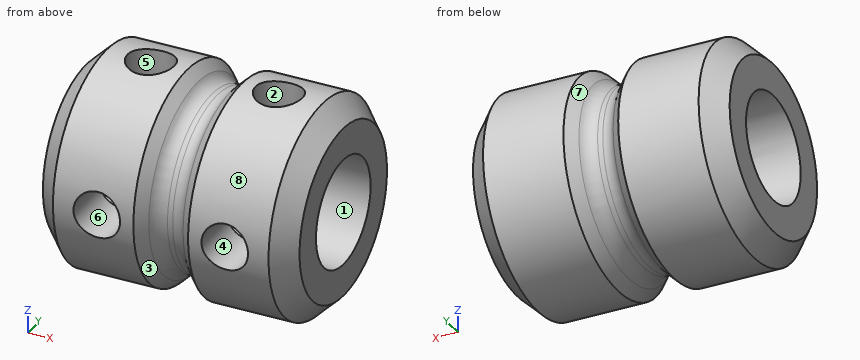
```python
from build123d import *

# Parameters (mm, degrees)
F0_R      = 7.874
F0_R_2    = 3.96875
F1_DEPTH  = 19.05
F2_SIZE2  = 1.524
F2_SIZE   = 1.524
F5_D      = 3.4544
F5_DEPTH  = 9.49325
F5_START  = 0.9537702
F5_TIP    = 1.0378064612
F8_D      = 3.4544
F8_DEPTH  = 9.4996
F8_START  = 0.9537702
F8_TIP    = 1.0378064612
F11_SIZE2 = 0.762
F11_SIZE  = 0.762


# Not quite as in the source:
# - a fillet or chamfer that OpenCascade refuses, or shapes differently, is made with other operations: its cross-section is extruded or revolved along the edge and cut away or added


with BuildPart() as f1:
    # F0 (on Right) → F1 (new body)
    with BuildSketch(Plane.YZ):
        Circle(F0_R)
        Circle(F0_R_2, mode=Mode.SUBTRACT)
    extrude(amount=F1_DEPTH)

    # F2
    f2_edges = [f1.edges().sort_by_distance(p)[0] for p in [
        (19.05, -7.874, 0),
        (0, -7.874, 0),
    ]]
    chamfer(f2_edges, length=F2_SIZE, length2=F2_SIZE2)

    # F5
    # its depths count from where the whole tool has entered the part; down to there all is cleared
    with Locations(Plane.XY.offset(8.636).offset(-F5_START)):
        with Locations((4.7752, 0), (14.2748, 0)):
            Hole(F5_D / 2, depth=F5_DEPTH)
            with Locations((0, 0, -(F5_DEPTH + F5_TIP / 2))):  # 118° drill point
                Cone(0, F5_D / 2, F5_TIP, mode=Mode.SUBTRACT)

    # F8
    # its depths count from where the whole tool has entered the part; down to there all is cleared
    with Locations(Plane.XZ.offset(8.636).offset(-F8_START)):
        with Locations((4.7752, 0), (14.2748, 0)):
            Hole(F8_D / 2, depth=F8_DEPTH)
            with Locations((0, 0, -(F8_DEPTH + F8_TIP / 2))):  # 118° drill point
                Cone(0, F8_D / 2, F8_TIP, mode=Mode.SUBTRACT)

    # F9 (on Front) → F10 (revolve, cut)
    with BuildSketch(Plane.XZ):
        Polygon((10.795, 8.9425863698), (9.525, 8.9425863698), (8.255, 8.9425863698), (8.255, 6.5122395754), (10.795, 6.5122395754), align=None)
    revolve(axis=Axis((-2.5821820018, 0, 0), (-1, 0, 0)), mode=Mode.SUBTRACT)

    # F11
    f11_edges = [f1.edges().sort_by_distance(p)[0] for p in [
        (8.255, -7.874, 0),
        (10.795, -7.874, 0),
    ]]
    chamfer(f11_edges, length=F11_SIZE, length2=F11_SIZE2)

    # F12: fillet of radius 1.27 on 2 edges, made by hand

    # F12_s1 → F12_t2 (revolve)
    with BuildSketch(Plane.XZ):
        with BuildLine():
            ThreePointArc((8.255, 7.112), (8.7166107711, 6.6722611385), (9.3337395013, 6.5122395754))
            Line((9.3337395013, 6.5122395754), (9.3337395013, 6.4868395754))
            Line((9.3337395013, 6.4868395754), (8.255, 6.4868395754))
            Line((8.255, 6.4868395754), (8.2296, 6.5122395754))
            ThreePointArc((8.2296, 6.5122395754), (8.2296, 6.8121197877), (8.23342521, 7.0985952085))
            Line((8.23342521, 7.0985952085), (8.255, 7.112))
        make_face()
    revolve(axis=Axis((8.255, 0, 0), (-1, 0, 0)))

    # F12_s3 → F12_t4 (revolve)
    with BuildSketch(Plane.XZ):
        with BuildLine():
            ThreePointArc((9.7162604987, 6.5122395754), (10.3333892289, 6.6722611385), (10.795, 7.112))
            Line((10.795, 7.112), (10.81657479, 7.0985952085))
            ThreePointArc((10.81657479, 7.0985952085), (10.8204, 6.8121197877), (10.8204, 6.5122395754))
            Line((10.8204, 6.5122395754), (10.795, 6.4868395754))
            Line((10.795, 6.4868395754), (9.7162604987, 6.4868395754))
            Line((9.7162604987, 6.4868395754), (9.7162604987, 6.5122395754))
        make_face()
    revolve(axis=Axis((10.795, 0, 0), (-1, 0, 0)))


solid = f1.part
```
Model file for the job. Use its own axes, mm. Face numbers are marked on the shaded views. A direction names the side the tool comes from. Give positions to 0.01 mm unless a question says otherwise; leave off trailing zeros. Order: outer loops, then holes, each group sorted by start corner. A loop starts at its lowest first (then second) coordinate and runs counter-clockwise, first axis right, second up.
1) 3-axis set-ups, long thin cutter, end or side, ignore diameter. For the marked faces 5, 6, 7 and 8: which of +Z, -Z, +X, -X, +Y, -Y reach the whole face in a straight line?
2) Saw through at A-A, the plane z = 0. Count the separate pieces of the cut face and the enclosed holes in it, then the cut area to 3 significant figures.
3) Mould opens along Z. For the marked faces 1, 2, 3 and 4 say: +Z half, -Z half, draft (parallel to the pull), parting line (faces both ways), or undercut.
4) Saw through at D-D, the plane x = 16.75. Write the cut outline in (y, z).
5) Pin check, flat tips, straight feed: pin 1 (1.5 mm diameter, centred on y = -6, z = -4, fed in from +X); pin 2 (5 mm diameter, centred on x = 16, z = 3.5, fed in from -Y); pin 3 (1 mm diameter, centred on x = 2, y = -1, fed in from +Z). Stop position of each tip, or through.
6) Saw through at C-C, the plane x = 14. Write the cut outline in (y, z), then the cut area to 3 significant figures.
7) Wall check: probe 1 along X at (y, z) = (0, 6.25); probe 2 along X at (y, z) = (-5.75, -0.75); probe 3 along Y at (x, z) = (10, 0). Give the ranges that are in metal, low to high.
Computed:
1. face 5: +Z
1. face 6: -Y
1. face 7: none
1. face 8: +X, -X
2. separate pieces: 4
2. enclosed holes: 0
2. area: 110 mm2
3. face 1: undercut
3. face 2: draft
3. face 3: parting line
3. face 4: undercut
4. outline: circle Ø15.75 at (0, 0); hole circle Ø7.94 at (0, 0)
5. pin 1: stops at x = 18.94
5. pin 2: stops at y = -7.81
5. pin 3: stops at z = 7.86
6. outline: (-7.69, -1.71) arc R7.87 ccw (long way) to (1.71, 7.69) - (1.71, 3.58) arc R3.97 cw (long way) to (-3.58, -1.71) - close; (-7.69, 1.71) - (-3.58, 1.71) arc R3.97 cw to (-1.71, 3.58) - (-1.71, 7.69) arc R7.87 ccw to start
6. area: 118 mm2
7. probe 1: x = 0 to 3.05, 6.5 to 12.55, 16 to 19.05
7. probe 2: x = 0 to 3.22, 6.33 to 12.72, 15.83 to 19.05
7. probe 3: y = -6.54 to -3.97, 3.97 to 6.54
